Autodesk Inventor part; units mm, degrees
ref_plane "YZ Plane" through (0, 0, 0) normal (1, 0, 0) x (0, 1, 0)
ref_plane "XZ Plane" through (0, 0, 0) normal (0, 1, 0) x (-1, 0, 0)
ref_plane "XY Plane" through (0, 0, 0) normal (0, 0, 1) x (1, 0, 0)
sketch "Sketch2" plane through (0, 0, 0) normal (1, 0, 0) x (0, 1, 0)
  line L0 (0, 21.8412) -> (4, 21.8412)
  line L1 (4, 21.8412) -> (4, 13.8412)
  line L2 (4, 13.8412) -> (6.5, 13.8412)
  line L3 (6.5, 13.8412) -> (6.5, 13.3412)
  line L4 (6.5, 13.3412) -> (4, 13.3412)
  line L5 (4, 13.3412) -> (4, -12.6588)
  line L6 (4, -12.6588) -> (0, -12.6588)
  line L7 (0, -12.6588) -> (0, 21.8412)
  point P0 (0, 0)
  dimension "d0" = 4
  dimension "d1" = 8
  dimension "d2" = 2.5
  dimension "d3" = 0.5
  dimension "d4" = 26
revolve "Revolution1" add sketch "Sketch2" angle 360 about axis through (0, 0, -12.6588) along (0, 0, 1)
sketch "Sketch3" plane through (0, 0, 21.8412) normal (0, 0, 1) x (1, 0, 0)
  line L0 (7.5, -1.3) -> (-7.5, -1.3)
  line L1 (-7.5, -1.3) -> (-7.5, 1.3)
  line L2 (-7.5, 1.3) -> (7.5, 1.3)
  line L3 (7.5, 1.3) -> (7.5, -1.3)
  circle A0 centre (0, 0) radius 4
  line L4 (7.5, -1.3) -> (-7.5, 1.3) construction
  line L5 (-7.5, -1.3) -> (7.5, 1.3) construction
  point P0 (3.7829, 1.3)
  point P1 (-3.7829, 1.3)
  point P2 (-3.7829, -1.3)
  point P3 (3.7829, -1.3)
  dimension "d14" = 2.6
  dimension "d15" = 15
extrude "Extrusion1" cut sketch "Sketch3" against normal blind 8 contours L0 A0 L2
sketch "Sketch5" plane through (-3.7829, -1.3, 21.8412) normal (0, 1, 0) x (1, 0, 0)
  circle A0 centre (3.7829, 4) radius 1.5
  line L0 (7.5657, 0) -> (0, 0)
  line L1 (7.5657, 0) -> (0, 0)
  line L2 (7.5657, 0) -> (0, 0)
  line L3 (7.5657, 8) -> (7.5657, 0)
  line L4 (7.5657, 0) -> (0, 0)
  line L5 (0, 0) -> (0, 8)
  line L6 (7.5657, 8) -> (0, 8)
  point P0 (3.7829, 21.8412)
  dimension "d8" = 4
  dimension "d9" = 3.7829
  dimension "d10" = 3.7829
  dimension "d13" = 3
extrude "Extrusion2" cut sketch "Sketch5" along normal through all both and the other way through all contours A0
equation "\"d9\" = d10"
properties part number "pole"
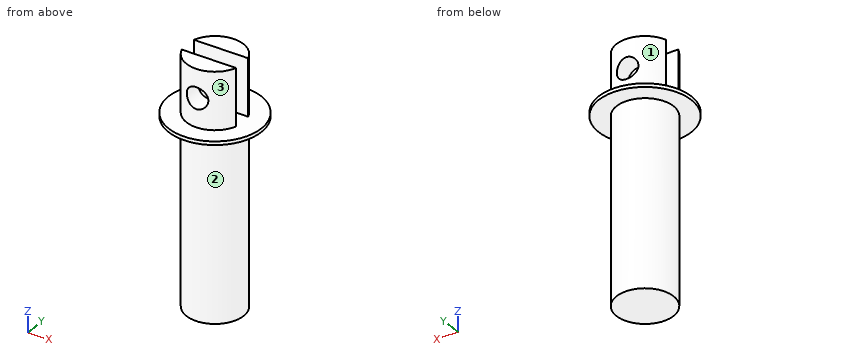
Source: CAD feature listing. Evaluate the final solid. Frame: model axes, mm. Face numbers are marked on the shaded views. A direction names the side the tool comes from. Give positions to 0.01 mm unless a question says otherwise; leave off trailing zeros. Write each loop counter-clockwise with the first axis right and the second up, starting at its lowest first coordinate (ties: lowest second). Pieces come first, ordered by that corner, then holes.
1. First-contact query: pin 1 (5 mm diameter, centred on x = 0, z = 17.84, fed in from -Y); pin 2 (1 mm diameter, centred on y = 2, z = 4.5, fed in from -X); pin 3 (2 mm diameter, centred on x = 4, y = -5, fed in from -Z). Flat tips, straight axial feed; report the tip coordinate or a pass-through.
2. Material intervals for line 1 along Z through (x, y) = (0, -1.75); line 2 along Z through (x, y) = (5.25, -1.75); line 3 along Y through (x, z) = (1.75, 15), sorted ascending.
3. Section query B-B (x = 0). Return the cut outline in (y, z).
4. Section query D-D (z = -10). Return the cut outline in (x, y), then the cut area to 3 significant figures.
5. Section query C-C (y = 0). Return the cut outline in (x, z).
6. Section query A-A (z = 17.5). Return the cut outline in (x, y).
7. Access query for the marked faces 1, 2 and 3. Directions: +Z, -Z, +X, -X, +Y, -Y. A direction counts if a zero-diameter tool reaches every point of the face in a straight line with its end or side. Return the directions, or none.
Output values:
1. pin 1: stops at y = -4
1. pin 2: stops at x = -3.71
1. pin 3: stops at z = 13.34
2. line 1: z = -12.66 to 16.34, 19.34 to 21.84
2. line 2: z = 13.34 to 13.84
2. line 3: y = -3.6 to -1.3, 1.3 to 3.6
3. outline: (-6.5, 13.34) - (-4, 13.34) - (-4, -12.66) - (4, -12.66) - (4, 13.34) - (6.5, 13.34) - (6.5, 13.84) - (4, 13.84) - (4, 16.34) - (1.3, 16.34) - (1.3, 13.84) - (-1.3, 13.84) - (-1.3, 16.34) - (-4, 16.34) - (-4, 13.84) - (-6.5, 13.84) - close; (-4, 19.34) - (-1.3, 19.34) - (-1.3, 21.84) - (-4, 21.84) - close; (1.3, 19.34) - (4, 19.34) - (4, 21.84) - (1.3, 21.84) - close
4. outline: circle Ø8 at (0, 0)
4. area: 50.3 mm2
5. outline: (-6.5, 13.34) - (-4, 13.34) - (-4, -12.66) - (4, -12.66) - (4, 13.34) - (6.5, 13.34) - (6.5, 13.84) - (-6.5, 13.84) - close
6. outline: (-3.78, -1.3) arc R4 ccw to (-1.46, -3.72) - (-1.46, -1.3) - close; (-3.78, 1.3) - (-1.46, 1.3) - (-1.46, 3.72) arc R4 ccw to start; (1.46, -3.72) arc R4 ccw to (3.78, -1.3) - (1.46, -1.3) - close; (1.46, 1.3) - (3.78, 1.3) arc R4 ccw to (1.46, 3.72) - close
7. face 1: +Z, +Y
7. face 2: -Z
7. face 3: +Z, -Y
